Geometry check sheet. Reference: drawing and pictorial views, mm from the part's lowest x, y, z. A direction names the side the tool comes from. Round coordinates to 2 decimals unless told otherwise and drop trailing zeros. Order: outer loops, then holes, each group sorted by start corner. A loop starts at its lowest first (then second) coordinate and runs counter-clockwise, first axis right, second up. Notation, with made-up numbers: (53, -12.5) -> (107, -12.5) arc R12 cw to (107, 7.5) -> close; hole circle Ø6 at (2, 32.5). An arc over 180 degrees is marked (long way). Put each result on its own line as item: value.
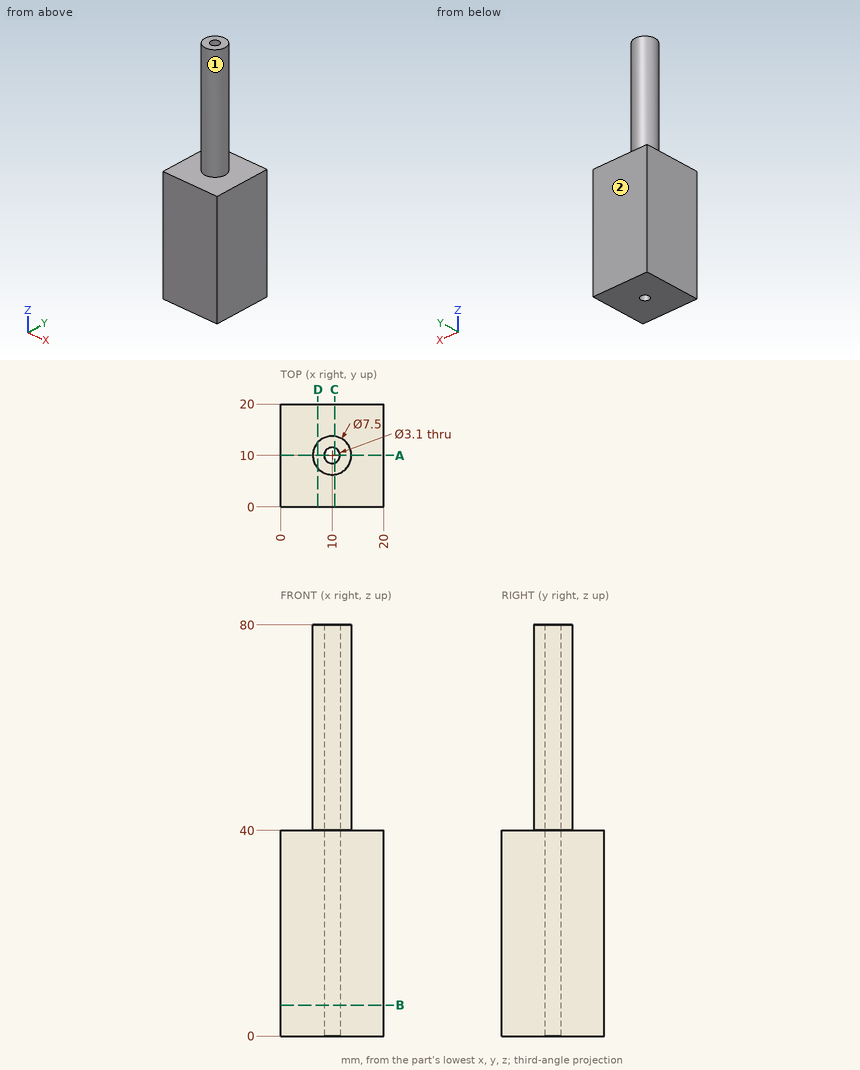
Item 1: Sectioned sample at B-B, the plane z = 6. Record the boundary of the cut face in (x, y), then the cut area to 3 significant figures.
Geometry check:
outline: (0, 0) -> (20, 0) -> (20, 20) -> (0, 20) -> close; hole circle Ø3.1 at (10, 10)
area: 392 mm2
Item 2: Tool access check on the marked faces 1 and 2. Record the directions out of +Z, -Z, +X, -X, +Y, -Y that give a thin tool (end or side, any length) a straight path to the whole face; none if there is none.
Geometry check:
face 1: +Z
face 2: +Z, -Z, +X, -X, +Y
Item 3: Material ranges on line 1 along Y through (x, z) = (10, 22.5); line 2 along Y through (x, z) = (10, 47.5); line 3 along Z through (x, y) = (5, 9.25), recorded low to high.
Geometry check:
line 1: 0 to 8.45, 11.55 to 20
line 2: 6.25 to 8.45, 11.55 to 13.75
line 3: 0 to 40
Item 4: Sectioned sample at A-A, the plane y = 10. Record the boundary of the cut face in (x, z).
Geometry check:
outline: (0, 0) -> (8.45, 0) -> (8.45, 80) -> (6.25, 80) -> (6.25, 40) -> (0, 40) -> close; (11.55, 0) -> (20, 0) -> (20, 40) -> (13.75, 40) -> (13.75, 80) -> (11.55, 80) -> close
Item 5: Sectioned sample at D-D, the plane x = 7.25. Record the boundary of the cut face in (y, z).
Geometry check:
outline: (0, 0) -> (20, 0) -> (20, 40) -> (12.55, 40) -> (12.55, 80) -> (7.45, 80) -> (7.45, 40) -> (0, 40) -> close
Item 6: Depth check by flat-ended pin: pin 1 Ø10 at (x, y) = (13.5, 12) entering from +Z; pin 2 Ø4 at (x, y) = (17.5, 9) entering from +Z; pin 3 Ø12 at (y, z) = (11.5, 71) entering from -X; pin 4 Ø4 at (y, z) = (5.5, 43.5) entering from -X. Enter the tip coordinate at first touch or a pass-through.
Geometry check:
pin 1: z = 80
pin 2: z = 40
pin 3: x = 6.25
pin 4: x = 7.2
Item 7: Sectioned sample at C-C, the plane x = 10.5. Record the boundary of the cut face in (y, z).
Geometry check:
outline: (0, 0) -> (8.53, 0) -> (8.53, 80) -> (6.28, 80) -> (6.28, 40) -> (0, 40) -> close; (11.47, 0) -> (20, 0) -> (20, 40) -> (13.72, 40) -> (13.72, 80) -> (11.47, 80) -> close
